Check sheet for the modelled part. Datum: model origin and axes. Units: mm. A direction names the side the tool comes from. Round coordinates to 2 decimals unless told otherwise and drop trailing zeros. Loops run counter-clockwise (first coordinate to the right, second up) from the corner with the lowest first, then second, coordinate; pieces in that order, holes last. Notation, with made-up numbers: (60.25, -36.75) - (115.25, -36.75) arc R17 ccw to (115.25, -26.75) - close; hole circle Ø9 at (41, -37). An arc over 180 degrees is marked (long way). Put each result on its own line as item: value.
```python
from build123d import *

# Parameters (mm, degrees)
PAD_DEPTH                 = 0.86
PAD002_DEPTH              = 0.86
FILLET_R                  = 2.2
FILLET001_R               = 1.9
CYLINDER_R                = 1.27
CYLINDER_DEPTH            = 10
BOX_W                     = 0.86
BOX_H                     = 12.57
BOX_DEPTH                 = 7.95
FILLET002_R               = 1.27
FILLET002_PLACEMENT_ANGLE = 180
CYLINDER001_R             = 1.27
CYLINDER001_DEPTH         = 10
BOX001_W                  = 0.86
BOX001_H                  = 12.57
BOX001_DEPTH              = 7.95
FILLET003_R               = 1.27
FILLET003_PLACEMENT_ANGLE = 180


with BuildPart() as body:
    # Sketch → Pad (new body)
    with BuildSketch(Plane.XZ):
        Polygon((0, 11.39), (4.12, 7.27), (4.12, 0), (14.31, 0), (14.31, 7.27), (18.42, 11.38), (18.42, 115.46), (19.95, 115.46), (21.59, 117.1), (21.59, 120.02), (2.54, 120.02), (2.54, 117.1), (0, 114.56), align=None)
    extrude(amount=PAD_DEPTH)


with BuildPart() as fillet001:
    # Sketch002 (on Face10 of Pad) → Pad002 (new body)
    with BuildSketch(Plane(origin=(0, 0, 120.02), x_dir=(-1, 0, 0), z_dir=(0, 0, 1))):
        Polygon((-21.59, 0.86), (-21.59, 3.73), (-16.21, 3.73), (-16.21, 8.15), (-21.59, 8.15), (-21.59, 12.29), (-13.97, 12.29), (-13.97, 8.1), (-10.92, 8.1), (-10.92, 12.29), (-2.54, 12.29), (-2.54, 0.86), align=None)
    extrude(amount=PAD002_DEPTH)


with BuildPart() as fillet001_1:
    # Body001 placement: moved
    add(fillet001.part.moved(Location((0, 0, -0.86))))

    # Fusion: union Body
    add(body.part)

    # Fillet
    fillet_edges = [fillet001_1.edges().sort_by_distance(p)[0] for p in [
        (16.21, -3.73, 119.59),
        (16.21, -8.15, 119.59),
    ]]
    fillet(fillet_edges, radius=FILLET_R)

    # Fillet001
    fillet001_edges = [fillet001_1.edges().sort_by_distance(p)[0] for p in [
        (4.12, -0.43, 0),
        (14.31, -0.43, 0),
    ]]
    fillet(fillet001_edges, radius=FILLET001_R)


with BuildPart() as cylinder:
    # Cylinder → Cylinder (new body)
    with BuildSketch(Plane(origin=(0, -9.4, 3.975), x_dir=(0, 0, -1), z_dir=(1, 0, 0))):
        Circle(CYLINDER_R)
    extrude(amount=CYLINDER_DEPTH)


with BuildPart() as fillet002:
    # Box → Box (new body)
    with BuildSketch(Plane(origin=(0, -12.57, 0), x_dir=(1, 0, 0), z_dir=(0, 0, 1))):
        with Locations((0.43, 6.285)):
            Rectangle(BOX_W, BOX_H)
    extrude(amount=BOX_DEPTH)

    # Cut: cut Cylinder
    add(cylinder.part, mode=Mode.SUBTRACT)

    # Fillet002
    fillet002_edges = [fillet002.edges().sort_by_distance(p)[0] for p in [
        (0.43, -12.57, 0),
        (0.43, -12.57, 7.95),
    ]]
    fillet(fillet002_edges, radius=FILLET002_R)


with BuildPart() as fillet002_1:
    # Fillet002 placement: moved
    add(fillet002.part.moved(Location((0.86, -0.86, 105.93))).rotate(Axis((0.86, -0.86, 105.93), (0, 0, 1)), FILLET002_PLACEMENT_ANGLE))


with BuildPart() as cylinder001:
    # Cylinder001 → Cylinder001 (new body)
    with BuildSketch(Plane(origin=(0, -9.4, 3.975), x_dir=(0, 0, -1), z_dir=(1, 0, 0))):
        Circle(CYLINDER001_R)
    extrude(amount=CYLINDER001_DEPTH)


with BuildPart() as obj1:
    # Box001 → Box001 (new body)
    with BuildSketch(Plane(origin=(0, -12.57, 0), x_dir=(1, 0, 0), z_dir=(0, 0, 1))):
        with Locations((0.43, 6.285)):
            Rectangle(BOX001_W, BOX001_H)
    extrude(amount=BOX001_DEPTH)

    # Cut001: cut Cylinder001
    add(cylinder001.part, mode=Mode.SUBTRACT)

    # Fillet003
    fillet003_edges = [obj1.edges().sort_by_distance(p)[0] for p in [
        (0.43, -12.57, 0),
        (0.43, -12.57, 7.95),
    ]]
    fillet(fillet003_edges, radius=FILLET003_R)


with BuildPart() as obj1_1:
    # Fillet003 placement: moved
    add(obj1.part.moved(Location((0.86, -0.86, 20.53))).rotate(Axis((0.86, -0.86, 20.53), (0, 0, 1)), FILLET003_PLACEMENT_ANGLE))

    # Fusion001: union Fillet001, Fillet002
    add(fillet001_1.part)
    add(fillet002_1.part)


solid = obj1_1.part
```
Item 1: Go/stop test with flat-tipped pins: pin 1 (4 mm diameter, centred on y = 4.5, z = 25.5, fed in from +X); pin 2 (6 mm diameter, centred on x = 9.5, z = 89.5, fed in from +Y); pin 3 (6.5 mm diameter, centred on x = 15.5, z = 81.5, fed in from -Y). Record where each tip stops, or that it passes through.
Filled sheet:
pin 1: x = 0.86
pin 2: y = 0
pin 3: y = -0.86
Item 2: Section check B-B on z = 47.5. Enter the section's corners in (x, y).
Filled sheet:
outline: (0, -0.86) - (18.42, -0.86) - (18.42, 0) - (0, 0) - close
Item 3: Section check C-C on y = -2.5. Enter the section's corners in (x, z), then the cut area to 3 significant figures.
Filled sheet:
outline: (2.54, 119.16) - (21.59, 119.16) - (21.59, 120.02) - (2.54, 120.02) - close
area: 16.4 mm²
Item 4: Release check for a two-part mould opening along Z. For faces 5 (the cylindrical face through (0.44, 7.28, 24.67)), 6 (the flat face through (12, -6, 120.02)), 7 (the cylindrical face through (4.662, -0.436, 0.571)), 8 (the cylindrical face through (0.436, 8.484, 111.174)) record: +Z half, -Z half, draft (parallel to the pull), parting line (faces both ways), or undercut.
Filled sheet:
face 5: undercut
face 6: +Z half
face 7: -Z half
face 8: undercut
Item 5: Section check A-A on y = 4.5. Enter the section's corners in (x, z), then the cut area to 3 significant figures.
Filled sheet:
outline: (0, 20.53) - (0.86, 20.53) - (0.86, 28.48) - (0, 28.48) - close; (0, 105.93) - (0.86, 105.93) - (0.86, 113.88) - (0, 113.88) - close
area: 13.7 mm²
Item 6: Thickness scan on line 1 (Y direction, x = 4, z = 99); line 2 (Z direction, x = 7, y = -5). Record the ranges inside material, lowest first. Write a range as from..to.
Filled sheet:
line 1: -0.86..0
line 2: 119.16..120.02
Item 7: Tool access check on faces 1 (the flat face through (2.54, -4.7, 119.6)), 2 (the flat face through (0.86, 6, 110)), 3 (the cylindrical face through (16.84, -4.39, 119.6)), 4 (the flat face through (12, -7, 119.16)). Record the directions out of +Z, -Z, +X, -X, +Y, -Y that give a thin tool (end or side, any length) a straight path to the whole face; none if there is none.
Filled sheet:
face 1: +Z, -X, +Y, -Y
face 2: +Z, -Z, +X, +Y
face 3: +Z, -Z, +X
face 4: -Z, +X, -X, -Y
